from build123d import *

# Parameters (mm, degrees)
T_LE_DE_BASE_PLI_E1_DEPTH             = 0.5
T_LE_PLI_E_SUR_AR_TE1_STRIP_W         = 3.4732
T_LE_PLI_E_SUR_AR_TE1_STRIP_H         = 0.5
T_LE_PLI_E_SUR_AR_TE1_STRIP_CUT_DEPTH = 171
T_LE_PLI_E_SUR_AR_TE1_DEPTH           = 171
PER_AGE1_START                        = -0.5
PER_AGE1_OUTLINE_R                    = 2.25
PER_AGE1_DEPTH                        = 0.5


# Read off the part's stored shape, not the designer's step: Perçage1
# Sheet-metal steps are written as plain solids
with BuildPart() as part:
    # Esquisse1 → Tôle de base pliée1 (new body)
    with BuildSketch(Plane.XY):
        Polygon((0, -85.5), (-17, -85.5), (-17, -78.5), (-10, -78.5), (-10, -73.5), (-17, -73.5), (-17, -59.5), (-10, -59.5), (-10, -54.5), (-17, -54.5), (-17, -40.5), (-10, -40.5), (-10, -35.5), (-17, -35.5), (-17, -21.5), (-10, -21.5), (-10, -16.5), (-17, -16.5), (-17, -2.5), (-10, -2.5), (-10, 2.5), (-17, 2.5), (-17, 16.5), (-10, 16.5), (-10, 21.5), (-17, 21.5), (-17, 35.5), (-10, 35.5), (-10, 40.5), (-17, 40.5), (-17, 54.5), (-10, 54.5), (-10, 59.5), (-17, 59.5), (-17, 73.5), (-10, 73.5), (-10, 78.5), (-17, 78.5), (-17, 85.5), (0, 85.5), align=None)
    extrude(amount=-T_LE_DE_BASE_PLI_E1_DEPTH)

    # Tôle pliée sur arête1 strip (across the edge) → Tôle pliée sur arête1 strip cut (cut)
    with BuildSketch(Plane(origin=(0, 85.5, -0.5), x_dir=(-1, 0, 0), z_dir=(0, -1, 0))):
        with Locations((-0.5, -0.25)):
            Rectangle(T_LE_PLI_E_SUR_AR_TE1_STRIP_W, T_LE_PLI_E_SUR_AR_TE1_STRIP_H)
    extrude(amount=T_LE_PLI_E_SUR_AR_TE1_STRIP_CUT_DEPTH, mode=Mode.SUBTRACT)

    # Tôle pliée sur arête1 section (across the edge) → Tôle pliée sur arête1 (add)
    with BuildSketch(Plane(origin=(0, 85.5, -0.5), x_dir=(-1, 0, 0), z_dir=(0, -1, 0))):
        with BuildLine():
            Line((0, 0.7366), (0, 17))
            Line((0, 17), (0.5, 17))
            Line((0.5, 17), (0.5, 0.7366))
            ThreePointArc((0.5, 0.7366), (0.715745145, 0.215745145), (1.2366, 0))
            Line((1.2366, 0), (1.2366, -0.5))
            ThreePointArc((1.2366, -0.5), (0.362191754, -0.137808246), (0, 0.7366))
        make_face()
    extrude(amount=T_LE_PLI_E_SUR_AR_TE1_DEPTH)

    # Perçage1 outline → Perçage1 (cut)
    with BuildSketch(Plane.YZ.offset(PER_AGE1_START)):
        with Locations((-70.5, -9.3683)):
            Circle(PER_AGE1_OUTLINE_R)
        with Locations((70.5, -9.3683)):
            Circle(PER_AGE1_OUTLINE_R)
    extrude(amount=PER_AGE1_DEPTH, mode=Mode.SUBTRACT)


solid = part.part
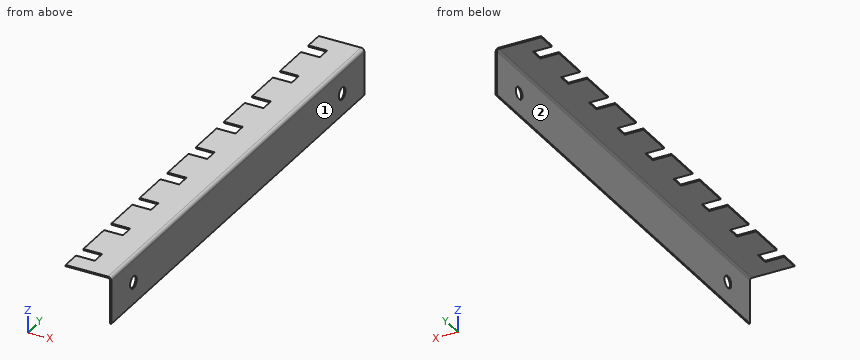
The model under review builds one solid part; all positions refer to its coordinate system, in mm. Face numbers are marked on the shaded views. A direction names the side the tool comes from. Round coordinates to 2 decimals unless told otherwise and drop trailing zeros. Write each loop counter-clockwise with the first axis right and the second up, starting at its lowest first coordinate (ties: lowest second). Pieces come first, ordered by that corner, then holes. Notation, with made-up numbers: M -29.75,9 L 2.25,9 A21 cw 2.25,28 Z; hole C -19.5,70.5 d4. An arc over 180 degrees is marked long. Use a Markdown table: item, result. Add a question column.
Q1. To check wall thickness, follow line 1 (Z direction, x = -0.25, y = 70.5); line 2 (Z direction, x = -5.5, y = 25). State the ranges of each line that lie inside material, in increasing order.
Q2. Machinability: for the marked faces 1 and 2, which of the approach directions +Z, -Z, +X, -X, +Y, -Y give a long, thin tool a straight path to every point of the face, cutting with its end or side? Answer none if there is none.
Q3. Insertion check: pin 1 (0.6 mm diameter, centred on y = 19, z = 0, fed in from -X); pin 2 (10 mm diameter, centred on x = -6, z = -7.5, fed in from +Y). Each pin has a flat end and moves straight along its axis. Give the tip position at first contact, or say it passes through.
Q4. We need section C-C, the plane z = -15. State the section outline as (x, y) points.
Q5. We need section A-A, the plane y = 70.5. State the section outline as (x, z) points, plus the area to 3 significant figures.
Q6. We need section D-D, the plane x = -12.5. Count the separate pieces of the cut face and the enclosed holes in it, plus the area to 3 significant figures.
Q7. We need section B-B, the plane y = -18.5. State the section outline as (x, z) points, plus the area to 3 significant figures.
Findings below:
| question | item | result |
|---|---|---|
| 1 | line 1 | z = -17.5 to -11.62, -7.12 to -0.49 |
| 1 | line 2 | z = -0.5 to 0 |
| 2 | face 1 | +Z, -Z, +X, +Y, -Y |
| 2 | face 2 | -Z, -X, +Y, -Y |
| 3 | pin 1 | stops at x = -10 |
| 3 | pin 2 | passes through |
| 4 | outline | M -0.5,-85.5 L 0,-85.5 L 0,85.5 L -0.5,85.5 Z |
| 5 | outline | M -17,-0.5 L -1.24,-0.5 A0.74 cw -0.5,-1.24 L -0.5,-7.12 L 0,-7.12 L 0,-1.24 A1.24 ccw -1.24,0 L -17,0 Z; M -0.5,-17.5 L 0,-17.5 L 0,-11.62 L -0.5,-11.62 Z |
| 5 | area | 14.5 mm² |
| 6 | separate pieces | 10 |
| 6 | enclosed holes | 0 |
| 6 | area | 63.0 mm² |
| 7 | outline | M -10,-0.5 L -1.24,-0.5 A0.74 cw -0.5,-1.24 L -0.5,-17.5 L 0,-17.5 L 0,-1.24 A1.24 ccw -1.24,0 L -10,0 Z |
| 7 | area | 13.3 mm² |
